Design review of the part built by this model. Coordinates are the model's own, in mm. A direction names the side the tool comes from. Round coordinates to 2 decimals unless told otherwise and drop trailing zeros. Write each loop counter-clockwise with the first axis right and the second up, starting at its lowest first coordinate (ties: lowest second). Pieces come first, ordered by that corner, then holes.
Autodesk Inventor part; units mm, degrees
ref_plane "cp1_XY" through (50.1015, 10.2235, 0) normal (1, 0, 0) x (0, 0, -1)
ref_plane "cp1_YZ" through (50.1015, 10.2235, 0) normal (0, 0, -1) x (0, 1, 0)
ref_plane "cp1_ZX" through (50.1015, 10.2235, 0) normal (0, 1, 0) x (1, 0, 0)
sketch "Sketch_1" plane through (0, 0, 0) normal (0, 0, 1) x (1, 0, 0)
  line L0 (100.203, 0) -> (0, 0)
  arc A0 (-0.6395, 9.3472) -> (-0.6395, 9.1676) centre (-0.5497, 9.2574) ccw
  line L1 (-0.6395, 9.1676) -> (-0.381, 8.9091)
  line L2 (-0.381, 8.9091) -> (0, 8.9091)
  line L3 (0, 8.9091) -> (0.762, 9.671)
  line L4 (0.762, 9.671) -> (99.441, 9.671)
  line L5 (99.441, 9.671) -> (100.203, 8.9091)
  line L6 (100.203, 8.9091) -> (100.584, 8.9091)
  line L7 (100.584, 8.9091) -> (100.8425, 9.1676)
  arc A1 (100.8425, 9.1676) -> (100.8425, 9.3472) centre (100.7527, 9.2574) ccw
  line L8 (100.8425, 9.3472) -> (100.1894, 10.0003)
  arc A2 (100.1894, 10.0003) -> (99.6505, 10.2235) centre (99.6506, 9.4615) ccw
  line L9 (99.6505, 10.2235) -> (0.5524, 10.2235)
  arc A3 (0.5524, 10.2235) -> (0.0136, 10.0003) centre (0.5524, 9.4615) ccw
  line L10 (0.0136, 10.0003) -> (-0.6395, 9.3472)
revolve "Revolution1" add sketch "Sketch_1" angle 360 about axis through (100.203, 0, 0) along (1, 0, 0)
sketch "Sketch_4" plane through (0, 0, 0) normal (0, 0, 1) x (1, 0, 0)
  circle A0 centre (8.763, 0) radius 1.1938
extrude "Extrusion1" cut sketch "Sketch_4" along normal blind 10.2235
ref_plane "cp1_XY" through (50.1015, 10.2235, 0) normal (1, 0, 0) x (0, 0, -1)
ref_plane "cp1_YZ" through (50.1015, 10.2235, 0) normal (0, 0, -1) x (0, 1, 0)
ref_plane "cp1_ZX" through (50.1015, 10.2235, 0) normal (0, 1, 0) x (1, 0, 0)
ref_plane "cp2_XY" through (50.1015, 0, -10.2235) normal (1, 0, 0) x (0, 0, -1)
ref_plane "cp2_YZ" through (50.1015, 0, -10.2235) normal (0, 0, -1) x (0, 1, 0)
ref_plane "cp2_ZX" through (50.1015, 0, -10.2235) normal (0, 1, 0) x (1, 0, 0)
ref_plane "cp3_XY" through (50.1015, -10.2235, 0) normal (1, 0, 0) x (0, 0, -1)
ref_plane "cp3_YZ" through (50.1015, -10.2235, 0) normal (0, 0, -1) x (0, 1, 0)
ref_plane "cp3_ZX" through (50.1015, -10.2235, 0) normal (0, 1, 0) x (1, 0, 0)
ref_plane "cp4_XY" through (50.1015, 0, 10.2235) normal (1, 0, 0) x (0, 0, -1)
ref_plane "cp4_YZ" through (50.1015, 0, 10.2235) normal (0, 0, -1) x (0, 1, 0)
ref_plane "cp4_ZX" through (50.1015, 0, 10.2235) normal (0, 1, 0) x (1, 0, 0)
ref_plane "tube_front_XY" through (0, 0, 0) normal (1, 0, 0) x (0, 0, -1)
ref_plane "tube_front_YZ" through (0, 0, 0) normal (0, 0, -1) x (0, 1, 0)
ref_plane "tube_front_ZX" through (0, 0, 0) normal (0, 1, 0) x (1, 0, 0)
ref_plane "tube_rear_XY" through (100.203, 0, 0) normal (1, 0, 0) x (0, 0, -1)
ref_plane "tube_rear_YZ" through (100.203, 0, 0) normal (0, 0, -1) x (0, 1, 0)
ref_plane "tube_rear_ZX" through (100.203, 0, 0) normal (0, 1, 0) x (1, 0, 0)
properties part number "04-3.9452C" material "Stainless Steel"
1) Add section A-A on y = 0. Count the separate pieces of the cut face and the enclosed holes in it, and give its area (3 significant figures).
2) Add section B-B on z = 0. State the section outline as (x, y) points.
3) For line 1 along Z through (x, y) = (33.5, 0); line 2 along Y through (x, z) = (54.5, -0.5); line 3 along Y through (x, z) = (15.5, 4.25), list the stretches that pass through material, from the lowest coordinate up.
4) Add section C-C on x = 83. State the section outline as (y, z) points, and give its area (3 significant figures).
5) For P1, Ø2, axis at x = 14, z = -7.5, coming from the -Y side; P2, Ø11.5, axis at y = 0, z = 0, coming from the +X side; P3, Ø2, axis at x = 8.763, y = 0, coming from the +Z side; P4, Ø4, axis at x = 43, z = 5, coming from the -Y side, all flat-tipped, find the tip position at first contact; note any pin that passes through.
6) For faces 3 (the face through (100.396, -1.931, -8.697)), 4 (the face through (9.9, -0.36, 9.91)), list the 3-axis set-ups (+Z, -Z, +X, -X, +Y, -Y) from which the entire face can be reached by the end or side of a thin tool; tool diameter is ignored.
7) The part is to be moulded in two halves that separate along Z. For faces 1 (the face through (49.408, -8.113, 6.221)), 2 (the face through (50.79, -2.1, -9.44)), say which applies: pulls with the +Z half, pulls with the -Z half, needs draft (parallel to the pull), parting line crosses it, or undercut.
Computed:
1. separate pieces: 3
1. enclosed holes: 0
1. area: 112 mm2
2. outline: (-0.64, -9.35) - (0.01, -10) arc R0.76 ccw to (0.55, -10.22) - (99.65, -10.22) arc R0.76 ccw to (100.19, -10) - (100.84, -9.35) arc R0.13 ccw to (100.84, -9.17) - (100.58, -8.91) - (100.2, -8.91) - (99.44, -9.67) - (0.76, -9.67) - (0, -8.91) - (-0.38, -8.91) - (-0.64, -9.17) arc R0.13 ccw to start; (-0.64, 9.17) - (-0.38, 8.91) - (0, 8.91) - (0.76, 9.67) - (99.44, 9.67) - (100.2, 8.91) - (100.58, 8.91) - (100.84, 9.17) arc R0.13 ccw to (100.84, 9.35) - (100.19, 10) arc R0.76 ccw to (99.65, 10.22) - (0.55, 10.22) arc R0.76 ccw to (0.01, 10) - (-0.64, 9.35) arc R0.13 ccw to start
3. line 1: z = -10.22 to -9.67, 9.67 to 10.22
3. line 2: y = -10.21 to -9.66, 9.66 to 10.21
3. line 3: y = -9.3 to -8.69, 8.69 to 9.3
4. outline: circle Ø20.45 at (0, 0); hole circle Ø19.34 at (0, 0)
4. area: 34.5 mm2
5. P1: stops at y = -7.89
5. P2: passes through
5. P3: stops at z = -9.62
5. P4: stops at y = -9.77
6. face 3: +X, -X
6. face 4: +Z
7. face 1: parting line crosses it
7. face 2: undercut
